from build123d import *

# Parameters (mm, degrees)
SKETCH1_W           = 1219.2
SKETCH1_H           = 749.3
BOSS_EXTRUDE1_DEPTH = 12.7
SKETCH2_W           = 1219.2
SKETCH2_H           = 749.3
SKETCH2_W_2         = 1193.8
SKETCH2_H_2         = 482.6
SKETCH2_R           = 5.08
BOSS_EXTRUDE2_DEPTH = 50.8
SKETCH3_R           = 6.35
CUT_EXTRUDE1_DEPTH  = 719.336294851


with BuildPart() as part:
    # Sketch1 → Boss-Extrude1 (new body)
    with BuildSketch(Plane.XY):
        Rectangle(SKETCH1_W, SKETCH1_H)
    extrude(amount=BOSS_EXTRUDE1_DEPTH)

    # Sketch2 → Boss-Extrude2 (add)
    with BuildSketch(Plane.XY.offset(12.7)):
        Rectangle(SKETCH2_W, SKETCH2_H)
        Rectangle(SKETCH2_W_2, SKETCH2_H_2, mode=Mode.SUBTRACT)
        with Locations(Location((495.3, -266.7, 0), (0, 0, 180))):
            Circle(SKETCH2_R, mode=Mode.SUBTRACT)
        with Locations(Location((406.4, -266.7, 0), (0, 0, 180))):
            Circle(SKETCH2_R, mode=Mode.SUBTRACT)
        with Locations(Location((-349.25, -342.9, 0), (0, 0, 180))):
            Circle(SKETCH2_R, mode=Mode.SUBTRACT)
        with Locations(Location((-349.25, -266.7, 0), (0, 0, 180))):
            Circle(SKETCH2_R, mode=Mode.SUBTRACT)
        with Locations(Location((-260.35, -342.9, 0), (0, 0, 180))):
            Circle(SKETCH2_R, mode=Mode.SUBTRACT)
        with Locations(Location((-260.35, -266.7, 0), (0, 0, 180))):
            Circle(SKETCH2_R, mode=Mode.SUBTRACT)
        with Locations(Location((406.4, -342.9, 0), (0, 0, 180))):
            Circle(SKETCH2_R, mode=Mode.SUBTRACT)
        with Locations(Location((495.3, -342.9, 0), (0, 0, 180))):
            Circle(SKETCH2_R, mode=Mode.SUBTRACT)
        with Locations((406.4, 342.9)):
            Circle(SKETCH2_R, mode=Mode.SUBTRACT)
        with Locations((495.3, 266.7)):
            Circle(SKETCH2_R, mode=Mode.SUBTRACT)
        with Locations((406.4, 266.7)):
            Circle(SKETCH2_R, mode=Mode.SUBTRACT)
        with Locations((495.3, 342.9)):
            Circle(SKETCH2_R, mode=Mode.SUBTRACT)
        with Locations((-260.35, 266.7)):
            Circle(SKETCH2_R, mode=Mode.SUBTRACT)
        with Locations((-349.25, 342.9)):
            Circle(SKETCH2_R, mode=Mode.SUBTRACT)
        with Locations((-349.25, 266.7)):
            Circle(SKETCH2_R, mode=Mode.SUBTRACT)
        with Locations((-260.35, 342.9)):
            Circle(SKETCH2_R, mode=Mode.SUBTRACT)
    extrude(amount=BOSS_EXTRUDE2_DEPTH)

    # Sketch3 → Cut-Extrude1 (cut, through all)
    with BuildSketch(Plane.XY.offset(63.5)):
        with Locations((-488.95, 311.15)):
            Circle(SKETCH3_R)
        with Locations((546.1, 323.85)):
            Circle(SKETCH3_R)
        with Locations(Location((546.1, -323.85, 0), (0, 0, 180))):
            Circle(SKETCH3_R)
        with Locations(Location((-488.95, -311.15, 0), (0, 0, 180))):
            Circle(SKETCH3_R)
    extrude(amount=-CUT_EXTRUDE1_DEPTH, mode=Mode.SUBTRACT)


solid = part.part
Verification items for the finished model (mm, model axes). A direction names the side the tool comes from. Coordinates: 2 decimals unless noted, no trailing zeros. Order: outer loops, then holes, each group sorted by start corner. A loop starts at its lowest first (then second) coordinate and runs counter-clockwise, first axis right, second up.
Item 1: Section check A-A, the plane z = 43.5. Give the number of separate pieces and of enclosed holes in the cut face, then the cut area to 3 significant figures.
Filled in:
separate pieces: 1
enclosed holes: 21
area: 336,000 mm2
Item 2: Material ranges on L1, parallel to X at y = -342.9, z = 45; L2, parallel to Y at x = -260, z = 36; L3, parallel to X at y = -266, z = 47, recorded low to high.
Filled in:
L1: x = -609.6 to -354.33, -344.17 to -265.43, -255.27 to 401.32, 411.48 to 490.22, 500.38 to 609.6
L2: y = -374.65 to -347.97, -337.83 to -271.77, -261.63 to -241.3, 241.3 to 261.63, 271.77 to 337.83, 347.97 to 374.65
L3: x = -609.6 to -354.28, -344.22 to -265.38, -255.32 to 401.37, 411.43 to 490.27, 500.33 to 609.6
Item 3: Access from +Z, -Z, +X, -X, +Y, -Y to the whole of each face (thin tool, end or side, straight path). Record for faces 1 (the face through (-9, 255, 63.5)), 2 (the face through (-8, -241.3, 38)).
Filled in:
face 1: +Z, +X, -X, +Y, -Y
face 2: +Z
Item 4: Section check C-C, the plane y = 187.5. Enter the section's corners in (x, z).
Filled in:
outline: (-609.6, 0) - (609.6, 0) - (609.6, 63.5) - (596.9, 63.5) - (596.9, 12.7) - (-596.9, 12.7) - (-596.9, 63.5) - (-609.6, 63.5) - close
Item 5: Section check B-B, the plane x = -401. Enter the section's corners in (y, z), then the cut area to 3 significant figures.
Filled in:
outline: (-374.65, 0) - (374.65, 0) - (374.65, 63.5) - (241.3, 63.5) - (241.3, 12.7) - (-241.3, 12.7) - (-241.3, 63.5) - (-374.65, 63.5) - close
area: 23,100 mm2
Item 6: Release check for a two-part mould opening along X. For faces 3 (the face through (609.6, -5, 31)), 4 (the face through (-8, 241.3, 38)), 5 (the face through (-8, 3, 12.7)), 6 (the face through (-9, -374.65, 31)) record: +X half, -X half, draft (parallel to the pull), parting line (faces both ways), or undercut.
Filled in:
face 3: +X half
face 4: undercut
face 5: undercut
face 6: draft
Item 7: Depth check by flat-ended pin: pin 1 (5 mm diameter, centred on x = -351, y = -265, fed in from +Z); pin 2 (10 mm diameter, centred on x = 546.1, y = -323.85, fed in from -Z). Enter the tip coordinate at first touch or a pass-through.
Filled in:
pin 1: stops at z = 12.7
pin 2: passes through
